Part model, mm, in its own coordinate system. Face numbers are marked on the shaded views. A direction names the side the tool comes from. Give positions to 0.01 mm unless a question says otherwise; leave off trailing zeros. Write each loop counter-clockwise with the first axis right and the second up, starting at its lowest first coordinate (ties: lowest second). Pieces come first, ordered by that corner, then holes. Notation, with made-up numbers: M -8.5,5 L 5.5,5 A31 ccw 5.5,30 Z; hole C 27,-30 d8. An arc over 180 degrees is marked long. Use CSV: the item, a comma, the result in double quotes. Start each with the question number.
Item 1: Which spindle directions (+Z, -Z, +X, -X, +Y, -Y) get a long thin tool onto all of the face, cutting with end or side? Do the marked faces 1, 2, 3 and 4. Say none if no direction does.
Item 2: Pin check, flat tips, straight feed: pin 1 (4.5 mm diameter, centred on x = 1, y = 20.5, fed in from +Z); pin 2 (1.5 mm diameter, centred on y = 22, z = 2, fed in from +X); pin 3 (3 mm diameter, centred on x = -1, y = 19, fed in from -Z). Stop position of each tip, or through.
Item 3: Cut at C-C (x = -1.25). List the corners of the cut face in (y, z).
Item 4: Cut at B-B (z = 1.75). List the corners of the cut face in (x, y).
Item 5: Mould opens along Z. For the marked faces 5, 6, 7 and 8 say: released by +Z, released by -Z, zero draft, split by the parting line, or undercut.
Item 6: Cut at D-D (y = 14.7). List the corners of the cut face in (x, z).
Item 7: Drill centre lines: line 1 (X direction, y = 18.5, z = -1); line 2 (Z direction, x = -1, y = 21.75); line 3 (X direction, y = 5.5, z = 0). Where is each one in solid material? Low to high. Write a range as [from, to].
Autodesk Inventor part; units mm, degrees
ref_plane "YZ Plane" through (0, 0, 0) normal (1, 0, 0) x (0, 1, 0)
ref_plane "XZ Plane" through (0, 0, 0) normal (0, 1, 0) x (-1, 0, 0)
ref_plane "XY Plane" through (0, 0, 0) normal (0, 0, 1) x (1, 0, 0)
sketch "Sketch1" plane through (0, 0, 0) normal (0, 1, 0) x (-1, 0, 0)
  line L0 (-3.95, -3.95) -> (3.95, -3.95)
  line L1 (3.95, -3.95) -> (3.95, 3.95)
  line L2 (3.95, 3.95) -> (-3.95, 3.95)
  line L3 (-3.95, 3.95) -> (-3.95, -3.95)
  line L4 (-3.95, -3.95) -> (3.95, 3.95) construction
  line L5 (3.95, -3.95) -> (-3.95, 3.95) construction
  point P0 (0, 0)
  dimension "d0" = 7.9
  dimension "d1" = 7.9
extrude "Extrusion1" add sketch "Sketch1" along normal blind 24.6
sketch "Sketch2" plane through (-3.95, 0, 3.95) normal (0, 0, 1) x (1, 0, 0)
  line L0 (7.9, 0) -> (7.9, 24.6)
  line L1 (0, 24.6) -> (7.9, 24.6)
  line L2 (0, 0) -> (0, 24.6)
  circle A0 centre (0, 14.7) radius 1.3
  circle A1 centre (7.9, 14.7) radius 1.3
  point P0 (3.95, 0)
  dimension "d4" = 2.6
  dimension "d5" = 2.6
  dimension "d6" = 9.9
  dimension "d7" = 9.9
extrude "Extrusion2" cut sketch "Sketch2" against normal through all
sketch "Sketch3" plane through (0, 0, 0) normal (0, -1, 0) x (1, 0, 0)
  line L0 (-2.5, -2.5) -> (2.5, -2.5)
  line L1 (2.5, -2.5) -> (2.5, 2.5)
  line L2 (2.5, 2.5) -> (-2.5, 2.5)
  line L3 (-2.5, 2.5) -> (-2.5, -2.5)
  line L4 (-2.5, -2.5) -> (2.5, 2.5) construction
  line L5 (2.5, -2.5) -> (-2.5, 2.5) construction
  point P0 (0, 0)
  dimension "d10" = 5
  dimension "d11" = 5
extrude "Extrusion3" cut sketch "Sketch3" against normal blind 15
sketch "Sketch4" plane through (0, 24.6, 0) normal (0, 1, 0) x (1, 0, 0)
  line L0 (-3.95, 3.95) -> (-3.95, -3.95)
  line L1 (-3.95, -3.95) -> (3.95, -3.95)
  line L2 (3.95, -3.95) -> (3.95, 3.95)
  line L3 (-3.95, 0) -> (-2.95, 0)
  line L4 (-2.95, 0) -> (-2.95, -2.95)
  line L5 (-2.95, -2.95) -> (2.95, -2.95)
  line L6 (2.95, -2.95) -> (2.95, 0)
  line L7 (2.95, 0) -> (3.95, 0)
  point P0 (0, 0)
  dimension "d14" = 1
  dimension "d15" = 1
  dimension "d16" = 1
extrude "Extrusion4" cut sketch "Sketch4" against normal blind 8
sketch "Sketch5" plane through (0, 24.6, 0) normal (0, 1, 0) x (1, 0, 0)
  line L0 (3.95, 3.95) -> (-3.95, 3.95)
  line L1 (-3.95, 3.95) -> (-3.95, 0)
  line L2 (-2.95, 2.95) -> (2.95, 2.95)
  line L3 (2.95, 2.95) -> (2.95, 0)
  line L4 (2.95, 0) -> (-2.95, 0)
  line L5 (-2.95, 0) -> (-2.95, 2.95)
  line L6 (-2.95, 2.95) -> (2.95, 0) construction
  line L7 (2.95, 2.95) -> (-2.95, 0) construction
  point P0 (0, 0)
  point P1 (0, 1.475)
  dimension "d19" = 1
  dimension "d20" = 1
extrude "Extrusion5" cut sketch "Sketch5" against normal blind 8
sketch "Sketch6" plane through (0, 0, 0) normal (0, -1, 0) x (1, 0, 0)
  line L0 (3.95, -3.95) -> (-3.95, -3.95)
  line L1 (3.95, 3.95) -> (3.95, -3.95)
  line L2 (-3.95, -3.95) -> (-3.95, 3.95)
  line L3 (1.5, -4.45) -> (-1.5, -4.45)
  line L4 (1.5, -4.45) -> (1, -3.95)
  line L5 (-1.5, -4.45) -> (-1, -3.95)
  line L6 (3.95, -3.95) -> (2.5, -2.5) construction
  line L7 (4.45, -1.5) -> (4.45, 1.5)
  line L8 (4.45, -1.5) -> (3.95, -1)
  line L9 (4.45, 1.5) -> (3.95, 1)
  line L10 (3.95, 1) -> (3.95, -1)
  point P0 (0, 0)
  dimension "d23" = 3
  dimension "d24" = 1.5
  dimension "d26" = 0.5
  dimension "d27" = 45
  dimension "d28" = 45
extrude "Extrusion6" add sketch "Sketch6" against normal blind 12
sketch "Sketch7" plane through (0, 0, 0) normal (0, -1, 0) x (1, 0, 0)
  line L0 (-2.5, -2.5) -> (-2.5, 2.5)
  line L1 (-3.95, -3.95) -> (-3.95, 3.95)
  line L2 (-1.5, -4.45) -> (1.5, -4.45)
  line L3 (1.5, -4.45) -> (1, -3.95)
  line L4 (-3.95, -1) -> (-3.45, -1.5)
  line L5 (-3.45, -1.5) -> (-3.45, 1.5)
  line L6 (-3.45, 1.5) -> (-3.95, 1)
  line L7 (-3.95, 1) -> (-3.95, -1)
  line L8 (-3.95, 3.95) -> (-2.5, 2.5) construction
  line L9 (1, 3.95) -> (1.5, 3.45)
  line L10 (1.5, 3.45) -> (-1.5, 3.45)
  line L11 (-1.5, 3.45) -> (-1, 3.95)
  line L12 (-1, 3.95) -> (1, 3.95)
  point P0 (0, 0)
  dimension "d34" = 3
  dimension "d35" = 1.5
  dimension "d36" = 0.5
extrude "Extrusion7" cut sketch "Sketch7" against normal blind 12
properties part number "PowerPole45" material "ABS Plastic"
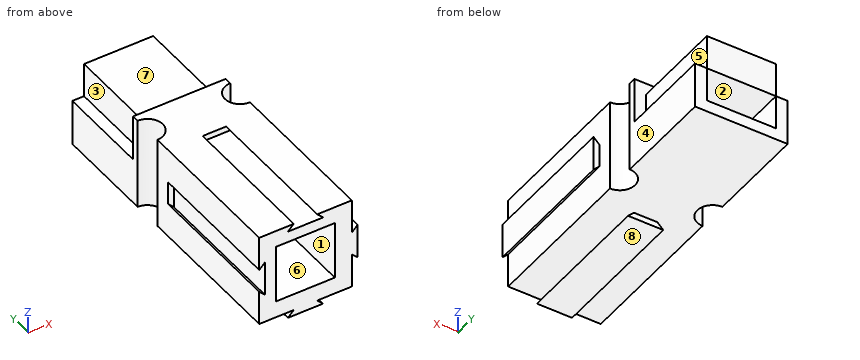
Worked answers:
1,face 1,"-Y"
1,face 2,"+Y"
1,face 3,"+Z, -X, +Y"
1,face 4,"+Z, -Z, +X, +Y"
2,pin 1,"stops at z = 2.95"
2,pin 2,"stops at x = 2.95"
2,pin 3,"stops at z = -3.95"
3,outline,"M 0,-4.45 L 12,-4.45 L 12,-4.2 L 0,-4.2 Z; M 0,-3.95 L 24.6,-3.95 L 24.6,-2.95 L 16.6,-2.95 L 16.6,0 L 24.6,0 L 24.6,2.95 L 16.6,2.95 L 16.6,3.95 L 0,3.95 L 0,3.7 L 12,3.7 L 12,3.45 L 0,3.45 L 0,2.5 L 15,2.5 L 15,-2.5 L 0,-2.5 Z"
4,outline,"M -3.95,0 L -2.5,0 L -2.5,15 L 2.5,15 L 2.5,0 L 3.95,0 L 3.95,13.4 A1.3 cw 3.95,16 L 3.95,16.6 L 2.95,16.6 L 2.95,24.6 L -2.95,24.6 L -2.95,16.6 L -3.95,16.6 L -3.95,16 A1.3 cw -3.95,13.4 Z"
5,face 5,"zero draft"
5,face 6,"undercut"
5,face 7,"released by +Z"
5,face 8,"released by -Z"
6,outline,"M -2.65,-3.95 L 2.65,-3.95 L 2.65,3.95 L -2.65,3.95 Z; hole M -2.5,-2.5 L 2.5,-2.5 L 2.5,2.5 L -2.5,2.5 Z"
7,line 1,"x = [-3.95, -2.95], [2.95, 3.95]"
7,line 2,"z = [-3.95, -2.95], [0, 2.95]"
7,line 3,"x = [-3.45, -2.5], [2.5, 4.45]"
